Check sheet for the modelled part. Datum: model origin and axes. Units: mm. Give positions to 0.01 mm unless a question says otherwise; leave off trailing zeros. Order: outer loops, then holes, each group sorted by start corner. A loop starts at its lowest first (then second) coordinate and runs counter-clockwise, first axis right, second up.
```python
from build123d import *

# Parameters (mm, degrees)
SKETCH1_R           = 25
BOSS_EXTRUDE1_DEPTH = 3
SKETCH6_R           = 1
CUT_EXTRUDE3_DEPTH  = 3
SKETCH7_R           = 1.35
CUT_EXTRUDE4_DEPTH  = 3
SKETCH10_W          = 6
SKETCH10_H          = 3
SKETCH10_W_2        = 3
SKETCH10_H_2        = 6
CUT_EXTRUDE5_DEPTH  = 3


with BuildPart() as part:
    # Sketch1 → Boss-Extrude1 (new body)
    with BuildSketch(Plane.XY):
        Circle(SKETCH1_R)
    extrude(amount=BOSS_EXTRUDE1_DEPTH)

    # Sketch6 → Cut-Extrude3 (cut)
    with BuildSketch(Plane.XY.offset(3)):
        with Locations((0, 23)):
            Circle(SKETCH6_R)
        with Locations((3.27324128, 22.765893163)):
            Circle(SKETCH6_R)
        with Locations((6.479848807, 22.068338393)):
            Circle(SKETCH6_R)
        with Locations((9.554545299, 20.921535893)):
            Circle(SKETCH6_R)
        with Locations((12.434738801, 19.348831255)):
            Circle(SKETCH6_R)
        with Locations((15.061796881, 17.38224021)):
            Circle(SKETCH6_R)
        with Locations((17.38224021, 15.061796881)):
            Circle(SKETCH6_R)
        with Locations((19.348831255, 12.434738801)):
            Circle(SKETCH6_R)
        with Locations((20.921535893, 9.554545299)):
            Circle(SKETCH6_R)
        with Locations((22.068338393, 6.479848807)):
            Circle(SKETCH6_R)
        with Locations((22.765893163, 3.27324128)):
            Circle(SKETCH6_R)
        with Locations((23, 0)):
            Circle(SKETCH6_R)
        with Locations((22.765893163, -3.27324128)):
            Circle(SKETCH6_R)
        with Locations((22.068338393, -6.479848807)):
            Circle(SKETCH6_R)
        with Locations((20.921535893, -9.554545299)):
            Circle(SKETCH6_R)
        with Locations((19.348831255, -12.434738801)):
            Circle(SKETCH6_R)
        with Locations((17.38224021, -15.061796881)):
            Circle(SKETCH6_R)
        with Locations((15.061796881, -17.38224021)):
            Circle(SKETCH6_R)
        with Locations((12.434738801, -19.348831255)):
            Circle(SKETCH6_R)
        with Locations((9.554545299, -20.921535893)):
            Circle(SKETCH6_R)
        with Locations((6.479848807, -22.068338393)):
            Circle(SKETCH6_R)
        with Locations((3.27324128, -22.765893163)):
            Circle(SKETCH6_R)
        with Locations((0, -23)):
            Circle(SKETCH6_R)
        with Locations((-3.27324128, -22.765893163)):
            Circle(SKETCH6_R)
        with Locations((-6.479848807, -22.068338393)):
            Circle(SKETCH6_R)
        with Locations((-9.554545299, -20.921535893)):
            Circle(SKETCH6_R)
        with Locations((-12.434738801, -19.348831255)):
            Circle(SKETCH6_R)
        with Locations((-15.061796881, -17.38224021)):
            Circle(SKETCH6_R)
        with Locations((-17.38224021, -15.061796881)):
            Circle(SKETCH6_R)
        with Locations((-19.348831255, -12.434738801)):
            Circle(SKETCH6_R)
        with Locations((-20.921535893, -9.554545299)):
            Circle(SKETCH6_R)
        with Locations((-22.068338393, -6.479848807)):
            Circle(SKETCH6_R)
        with Locations((-22.765893163, -3.27324128)):
            Circle(SKETCH6_R)
        with Locations((-23, 0)):
            Circle(SKETCH6_R)
        with Locations((-22.765893163, 3.27324128)):
            Circle(SKETCH6_R)
        with Locations((-22.068338393, 6.479848807)):
            Circle(SKETCH6_R)
        with Locations((-20.921535893, 9.554545299)):
            Circle(SKETCH6_R)
        with Locations((-19.348831255, 12.434738801)):
            Circle(SKETCH6_R)
        with Locations((-17.38224021, 15.061796881)):
            Circle(SKETCH6_R)
        with Locations((-15.061796881, 17.38224021)):
            Circle(SKETCH6_R)
        with Locations((-12.434738801, 19.348831255)):
            Circle(SKETCH6_R)
        with Locations((-9.554545299, 20.921535893)):
            Circle(SKETCH6_R)
        with Locations((-6.479848807, 22.068338393)):
            Circle(SKETCH6_R)
        with Locations((-3.27324128, 22.765893163)):
            Circle(SKETCH6_R)
    extrude(amount=-CUT_EXTRUDE3_DEPTH, mode=Mode.SUBTRACT)

    # Sketch7 → Cut-Extrude4 (cut)
    with BuildSketch(Plane.XY.offset(3)):
        Circle(SKETCH7_R)
    extrude(amount=-CUT_EXTRUDE4_DEPTH, mode=Mode.SUBTRACT)

    # Sketch10 → Cut-Extrude5 (cut)
    with BuildSketch(Plane.XY.offset(3)):
        with Locations((0, 7.5)):
            Rectangle(SKETCH10_W, SKETCH10_H)
        with Locations((7.5, 0)):
            Rectangle(SKETCH10_W_2, SKETCH10_H_2)
        with Locations((0, -7.5)):
            Rectangle(SKETCH10_W, SKETCH10_H)
        with Locations((-7.5, 0)):
            Rectangle(SKETCH10_W_2, SKETCH10_H_2)
    extrude(amount=-CUT_EXTRUDE5_DEPTH, mode=Mode.SUBTRACT)


solid = part.part
```
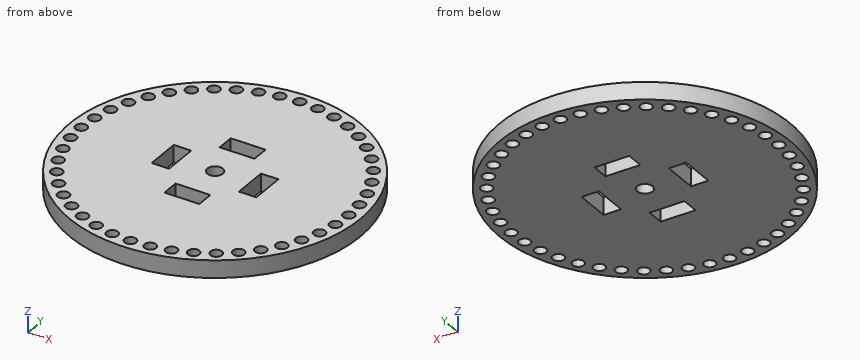
Q1. Sectioned sample at A-A, the plane y = 0. Record the cut outline in (x, z).
Q2. Go/stop test with flat-tipped pins: P1, Ø0.9, axis at y = -7.5, z = 1, coming from the -X side; P2, Ø0.9, axis at x = 7.5, z = 2, coming from the +Y side; P3, Ø1, axis at x = 17.5, z = 1, coming from the -Y side. Record where each tip stops, or that it passes through.
Q3. Material ranges on line 1 (X direction, y = -6.5, z = 2.75); line 2 (X direction, y = -21, z = 0.5); line 3 (X direction, y = -4, z = 0.85), recorded low to high.
Q4. Sectioned sample at B-B, the plane z = 2.2. Count the separate pieces of the cut face and the enclosed holes in it, plus the area to 3 significant figures.
Filled in:
1. outline: (-25, 0) - (-24, 0) - (-24, 3) - (-25, 3) - close; (-22, 0) - (-9, 0) - (-9, 3) - (-22, 3) - close; (-6, 0) - (-1.35, 0) - (-1.35, 3) - (-6, 3) - close; (1.35, 0) - (6, 0) - (6, 3) - (1.35, 3) - close; (9, 0) - (22, 0) - (22, 3) - (9, 3) - close; (24, 0) - (25, 0) - (25, 3) - (24, 3) - close
2. P1: stops at x = -23.99
2. P2: stops at y = 23.99
2. P3: stops at y = -18.33
3. line 1: x = -24.14 to -23.07, -21.07 to -3, 3 to 21.07, 23.07 to 24.14
3. line 2: x = -13.56 to -10.55, -8.56 to 8.56, 10.55 to 13.56
3. line 3: x = -24.68 to -23.45, -22.08 to 22.08, 23.45 to 24.68
4. separate pieces: 1
4. enclosed holes: 49
4. area: 1,750 mm2
